Source: CAD feature listing. Evaluate the final solid. Frame: model axes, mm. Face numbers are marked on the shaded views. A direction names the side the tool comes from. Round coordinates to 2 decimals unless told otherwise and drop trailing zeros. Write each loop counter-clockwise with the first axis right and the second up, starting at its lowest first coordinate (ties: lowest second). Pieces come first, ordered by that corner, then holes. Notation, with made-up numbers: M -23.5,-6 L -16.5,-6 A20 ccw -16.5,11 Z; hole C 9,71 d4. An arc over 180 degrees is marked long. Answer in a Markdown table with one row per item. Add a question column.
Item 1: Cut plane A-A on x = -2.5. Return loops of the section in (y, z), and give its area (3 significant figures).
Item 2: Mould query, pull axis X, two halves, no side actions, for the marked faces 5, 6 and 7. Classes: released by +X, released by -X, zero draft, split by the parting line, or undercut.
Item 3: Cut plane C-C on z = 4.25. Return loops of the section in (x, y), and give its area (3 significant figures).
Item 4: Contact query for flat-ended pins moving along their axis: pin 1 (3 mm diameter, centred on x = -1.5, y = 0.5, fed in from +Z); pin 2 (1.5 mm diameter, centred on x = 1, y = 0, fed in from -Z); pin 3 (1.5 mm diameter, centred on y = 7.5, z = 2, fed in from -X); pin 4 (1.7 mm diameter, centred on y = -4.5, z = 2, fed in from -X). Output: stop coordinate, or through.
Item 5: Set-up query: the marked faces 1, 2, 3 and 4. Return all of +Z, -Z, +X, -X, +Y, -Y with unobstructed straight access to the full face (end or side cutting, diameter ignored); none if empty.
Item 6: Material intervals for probe 1 along X at (y, z) = (2.5, 0.9); probe 2 along Z at (x, y) = (-1.5, -7.75); probe 3 along X at (y, z) = (5, 1.15), sorted ascending.
Item 7: Cut plane B-B on y = 0.25. Return loops of the section in (x, z).
Autodesk Inventor part; units mm, degrees
ref_plane "YZ Plane" through (0, 0, 0) normal (1, 0, 0) x (0, 1, 0)
ref_plane "XZ Plane" through (0, 0, 0) normal (0, 1, 0) x (-1, 0, 0)
ref_plane "XY Plane" through (0, 0, 0) normal (0, 0, 1) x (1, 0, 0)
sketch "Schizzo1" plane through (0, 0, 0) normal (0, 0, 1) x (1, 0, 0)
  line L0 (-7, 10) -> (7, 10)
  line L1 (7, 10) -> (7, -10)
  line L2 (7, -10) -> (-7, -10)
  line L3 (-7, -10) -> (-7, 10)
  line L4 (-7, 10) -> (7, -10) construction
  line L5 (7, 10) -> (-7, -10) construction
  line L6 (-5.5, 10) -> (-5.5, -10)
  line L7 (5.5, 10) -> (5.5, -10)
  line L8 (-7, 6) -> (-5.5, 6)
  line L9 (-7, 4) -> (-5.5, 4)
  line L10 (-7, -4) -> (-5.5, -4)
  line L11 (-7, -6) -> (-5.5, -6)
  line L12 (-7, 6) -> (-7.5, 6)
  line L13 (-7.5, 6) -> (-7.5, 4)
  line L14 (-7.5, 4) -> (-7, 4)
  line L15 (-7, 4) -> (-7, 6)
  line L16 (-7, -4) -> (-7.5, -4)
  line L17 (-7.5, -4) -> (-7.5, -6)
  line L18 (-7.5, -6) -> (-7, -6)
  line L19 (-7, -6) -> (-7, -4)
  point P0 (0, 0)
  point P1 (0, 0)
  point P2 (-6.25, 4)
  point P3 (-6.25, -6)
  point P4 (-7, 5)
  dimension "d0" = 14
  dimension "d1" = 20
  dimension "d2" = 1.5
  dimension "d3" = 1.5
  dimension "d4" = 4
  dimension "d5" = 2
  dimension "d6" = 2
  dimension "d7" = 4
  dimension "d19" = 0.5
extrude "Estrusione1" add sketch "Schizzo1" along normal blind 1 contours L0 L6 L8 L3 | L0 L7 L2 L6 | L8 L6 L9 L3 | L0 L1 L2 L7 | L9 L6 L10 L3 | L10 L6 L11 L3 | L2 L3 L11 L6
extrude "Estrusione2" add sketch "Schizzo1" along normal blind 4.5 contours L0 L1 L2 L7
extrude "Estrusione3" add sketch "Schizzo1" along normal blind 5.5 contours L8 L6 L9 L3 | L10 L6 L11 L3
sketch "Schizzo2" plane through (-5.5, 4, 1) normal (1, 0, 0) x (0, 0, -1)
  line L0 (0, -10) -> (-4.5, -10)
  line L1 (-3, -10) -> (-3, -8)
  line L2 (0, -8) -> (-4.5, -8)
  line L3 (0, 0) -> (-4.5, 0)
  line L4 (-3, 0) -> (-3, 2)
  line L5 (0, 2) -> (-4.5, 2)
  line L6 (-4.5, -10) -> (-4.5, -8)
  line L7 (-3, 0) -> (-4.5, 0)
  line L8 (-4.5, 0) -> (-4.5, 2)
  line L9 (-4.5, 2) -> (-3, 2)
  point P0 (1, -4)
  dimension "d14" = 1.5
extrude "Estrusione4" add sketch "Schizzo2" along normal blind 5
fillet "Raccordo1" radius 2 5 edges at (-6.25, -6, 1) (-6.25, -4, 1) (-6.25, 4, 1) (-6.25, 6, 1) (5.5, 0, 4.5)
fillet "Raccordo2" radius 0.75 8 edges at (-0.5, 5, 5.5) (-0.5, 5, 4) (-0.5, -5, 5.5) (-0.5, -5, 4) (-0.5, -6, 4.75) (-0.5, -4, 4.75) (-0.5, 4, 4.75) (-0.5, 6, 4.75)
extrude "Estrusione5" add sketch "Schizzo1" along normal blind 5.5 contours L3 L14 L13 L12 | L3 L18 L17 L16
sketch "Schizzo3" plane through (-7, -6, 3) normal (0, -1, 0) x (1, 0, 0)
  line L0 (-0.5, 2.5) -> (5.75, 2.5)
  line L1 (0.0105, 2.5) -> (-0.5, 2.5)
  line L2 (-0.5, 2.5) -> (-0.5, -3)
  line L3 (-0.5, -3) -> (0.0105, 2.5)
  point P0 (7, -3)
  point P1 (0.0105, 2.5)
extrude "Estrusione6" cut sketch "Schizzo3" against normal blind 90
fillet "Raccordo3" radius 0.5 1 edges at (-7.5, 5, 0)
equation "\"d0\" = Larghezza"
equation "\"d1\" = Lunghezza"
equation "\"d2\" = Parete"
equation "\"d3\" = d2"
equation "\"d4\" = Gancio_bordo"
equation "\"d7\" = d4"
equation "\"Lunghezza\" = 20"
equation "\"Larghezza\" = 14"
equation "\"Parete\" = 1.5"
equation "\"Gancio_gancio\" = 8"
equation "\"Gancio_bordo\" = 4"
equation "\"Gancio_larghezza_base\" = 2"
equation "\"Gancio_spessore\" = 1"
equation "\"Gancio_altezza\" = 5.5"
equation "\"Altezza_parete\" = 4.5"
equation "\"Spessore_base\" = 1"
equation "\"Gancio_larghezza\" = 1.5"
equation "\"Gancio_estrusione\" = 5"
properties part number "Supporto anello"
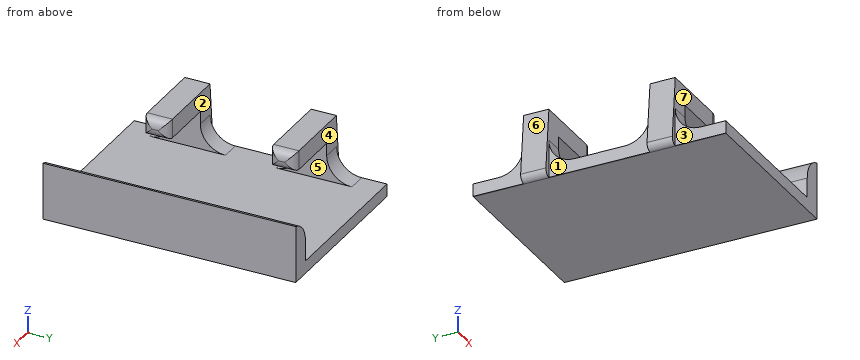
Results below:
| question | item | result |
|---|---|---|
| 1 | outline | M -10,0 L 10,0 L 10,1 L -10,1 Z; M -6,4 L -4,4 L -4,5.5 L -6,5.5 Z; M 4,4 L 6,4 L 6,5.5 L 4,5.5 Z |
| 1 | area | 26.0 mm2 |
| 2 | face 5 | undercut |
| 2 | face 6 | released by -X |
| 2 | face 7 | zero draft |
| 3 | outline | M -7.11,-6 L -1.25,-6 A0.75 ccw -0.69,-5.75 L -0.69,-4.25 A0.75 ccw -1.25,-4 L -7.11,-4 Z; M -7.11,4 L -1.25,4 A0.75 ccw -0.69,4.25 L -0.69,5.75 A0.75 ccw -1.25,6 L -7.11,6 Z; M 6.42,-10 L 7,-10 L 7,10 L 6.42,10 Z |
| 3 | area | 37.0 mm2 |
| 4 | pin 1 | z = 1 |
| 4 | pin 2 | z = 0 |
| 4 | pin 3 | x = 5.5 |
| 4 | pin 4 | x = -7.39 |
| 5 | face 1 | +Z, -Z, -X |
| 5 | face 2 | +Z, -X |
| 5 | face 3 | +Z, -Z, -X, -Y |
| 5 | face 4 | +Z, -X, +Y |
| 6 | probe 1 | -7 to 7 |
| 6 | probe 2 | 0 to 1 |
| 6 | probe 3 | -7.39 to -5.5, 5.5 to 7 |
| 7 | outline | M -7,0 A0.5 ccw -6.95,0 L 7,0 L 7,4.5 A2 ccw 5.5,2.56 L 5.5,1 L -7,1 Z |
